Can you work these out from the drawing? Everything is in mm from the part's minimum corner. Give positions to 0.01 mm unless a question says otherwise; leave off trailing zeros. Write each loop counter-clockwise with the first axis right and the second up, starting at its lowest first coordinate (ties: lowest second). Pieces come first, ordered by that corner, then holes. Notation, with made-up numbers: (78, -22) -> (117, -22) arc R16 ccw to (117, 5) -> close; hole circle Ø4 at (41.5, 50.25). An arc over 180 degrees is marked (long way). Write item = value, one per line. Start each with the question number.
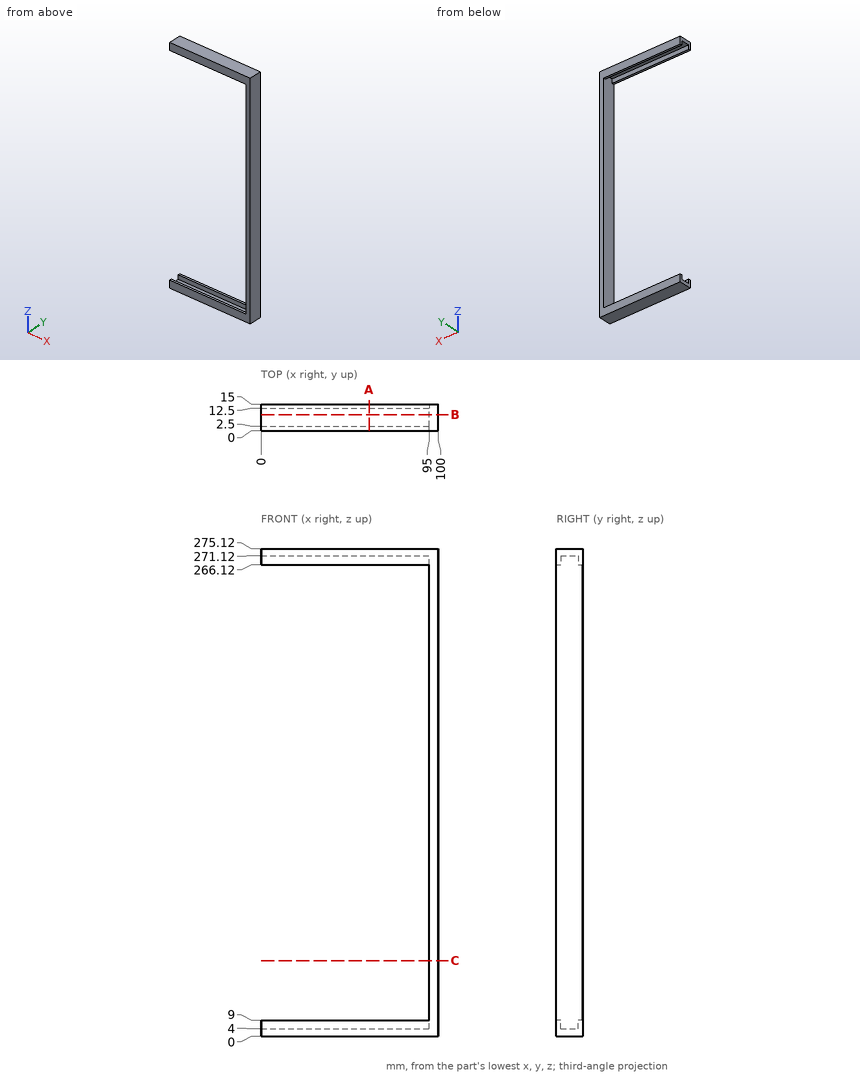
(1) I'm going to push a flat-ended pin straight in: pin 1 (7.5 mm diameter, centred on y = 7.5, z = 119, fed in from -X). Where does the tip first touch, or does it pass through?
(2) Imagine slicing it at A-A (x = 61). Please give me the cut outline in (y, z).
(3) Imagine slicing it at B-B (y = 9). Please give me the cut outline in (x, z), then the cut area to 3 significant figures.
(4) If I drill on line 1 along Z through (x, y) = (54.5, 1.75); line 2 along Z through (x, y) = (22, 11); line 3 along X through (y, z) = (10.5, 139), over which ranges is the centre line in solid material (lowest first)? Write a range as from..to.
(5) Imagine slicing it at C-C (z = 42.5). Please give me the cut outline in (x, y).
Answers below:
q1.pin_1 = 95
q2.outline = (0, 0) -> (15, 0) -> (15, 9) -> (12.5, 9) -> (12.5, 4) -> (2.5, 4) -> (2.5, 9) -> (0, 9) -> close; (0, 266.12) -> (2.5, 266.12) -> (2.5, 271.12) -> (12.5, 271.12) -> (12.5, 266.12) -> (15, 266.12) -> (15, 275.12) -> (0, 275.12) -> close
q3.outline = (0, 0) -> (100, 0) -> (100, 275.12) -> (0, 275.12) -> (0, 271.12) -> (95, 271.12) -> (95, 4) -> (0, 4) -> close
q3.area = 2,140 mm^2
q4.line_1 = 0..9, 266.12..275.12
q4.line_2 = 0..4, 271.12..275.12
q4.line_3 = 95..100
q5.outline = (95, 0) -> (100, 0) -> (100, 15) -> (95, 15) -> close
